from build123d import *

# Parameters (mm, degrees)
BOSS_EXTRUDE1_DEPTH      = 3.3734375
BOSS_EXTRUDE1_DEPTH_BACK = 3.3734375
SKETCH2_OUTSIDE_W        = 45.644
SKETCH2_OUTSIDE_H        = 47.608
SKETCH2_OUTSIDE_R        = 6.35
CUT_EXTRUDE1_DEPTH       = 7.746875
CUT_EXTRUDE1_TAPER       = 60
F_5_16_18_TAPPED_HOLE1_D = 6.5278


with BuildPart() as part:
    # Sketch1 → Boss-Extrude1 (new body, two sides)
    with BuildSketch(Plane(origin=(0, 0, 0), x_dir=(1, 0, 0), z_dir=(0, 1, 0))) as boss_extrude1_sk:
        Polygon((6.35, -3.666174209), (6.35, 3.666174209), (0, 7.332348419), (-6.35, 3.666174209), (-6.35, -3.666174209), (0, -7.332348419), align=None)
    extrude(amount=BOSS_EXTRUDE1_DEPTH)
    extrude(boss_extrude1_sk.sketch, amount=-BOSS_EXTRUDE1_DEPTH_BACK)

    # Sketch2 outside → Cut-Extrude1 (cut, through all)
    with BuildSketch(Plane(origin=(0, 3.3734375, 0), x_dir=(1, 0, 0), z_dir=(0, 1, 0))):
        Rectangle(SKETCH2_OUTSIDE_W, SKETCH2_OUTSIDE_H)
        Circle(SKETCH2_OUTSIDE_R, mode=Mode.SUBTRACT)
    cut_extrude1 = extrude(amount=-CUT_EXTRUDE1_DEPTH, taper=CUT_EXTRUDE1_TAPER, mode=Mode.SUBTRACT)

    # Mirror1: Cut-Extrude1 across plane
    add(cut_extrude1.mirror(Plane.ZX), mode=Mode.SUBTRACT)

    # 5/16-18 Tapped Hole1 (through all)
    with Locations(Plane(origin=(0, 3.3734375, 0), x_dir=(1, 0, 0), z_dir=(0, 1, 0))):
        with Locations((0, 0)):
            Hole(F_5_16_18_TAPPED_HOLE1_D / 2)


solid = part.part
Model file for the job. Use its own axes, mm. Give positions to 0.01 mm unless a question says otherwise; leave off trailing zeros. Loops run counter-clockwise (first coordinate to the right, second up) from the corner with the lowest first, then second, coordinate; pieces in that order, holes last.
Item 1: Slice it at A-A (y = -1.25). Write the cut outline in (x, z), plus the area to 3 significant figures.
Check values:
outline: (-6.35, -3.67) - (0, -7.33) - (6.35, -3.67) - (6.35, 3.67) - (0, 7.33) - (-6.35, 3.67) - close; hole circle Ø6.53 at (0, 0)
area: 106 mm2
Item 2: Drill centre lines: line 1 along X through (y, z) = (-2, 0.75); line 2 along Z through (x, y) = (1, -0.75) (3 decimals); line 3 along X through (y, z) = (-2.5, 1.5). Where is each one in solid material? Low to high.
Check values:
line 1: x = -6.35 to -3.18, 3.18 to 6.35
line 2: z = -6.755 to -3.107, 3.107 to 6.755
line 3: x = -6.35 to -2.9, 2.9 to 6.35
Item 3: Mould opens along Z. For faces 1 (the face through (5.698, -3.236, -3.308)), 2 (the face through (5.71, -3.24, 3.28)), 3 (the face through (-6.35, 0, 0)) say: +Z half, -Z half, draft (parallel to the pull), parting line (faces both ways), or undercut.
Check values:
face 1: -Z half
face 2: +Z half
face 3: draft
Item 4: Drop a flat-ended pin along its axis: P1, Ø1, axis at x = 1.5, y = 1, coming from the +Z side (3 decimals). Give the stop position or say it passes through.
Check values:
P1: stops at z = 6.755
